from build123d import *

# Parameters (mm, degrees)
SKETCH2_R           = 3.175
BOSS_EXTRUDE1_DEPTH = 57.15
SKETCH7_W           = 12.7
SKETCH7_H           = 15.875
CUT_EXTRUDE3_DEPTH  = 69.170141008
FILLET1_R           = 2.54


with BuildPart() as part:
    # Sketch2 → Boss-Extrude1 (new, symmetric)
    with BuildSketch(Plane(origin=(0, 0, 0), x_dir=(1, 0, 0), z_dir=(0, 1, 0))):
        with BuildLine():
            Line((-28.575, 6.35), (28.575, 6.35))
            ThreePointArc((28.575, 6.35), (34.925, 0), (28.575, -6.35))
            Line((28.575, -6.35), (-28.575, -6.35))
            ThreePointArc((-28.575, -6.35), (-34.925, 0), (-28.575, 6.35))
        make_face()
        with Locations(Location((28.575, 0, 0), (0, 0, 270))):
            Circle(SKETCH2_R, mode=Mode.SUBTRACT)
        with Locations(Location((-28.575, 0, 0), (0, 0, 270))):
            Circle(SKETCH2_R, mode=Mode.SUBTRACT)
    extrude(amount=BOSS_EXTRUDE1_DEPTH, both=True)

    # Sketch7 → Cut-Extrude3 (cut, through all)
    with BuildSketch(Plane.XY.offset(6.35)):
        with Locations((0, 49.2125)):
            Rectangle(SKETCH7_W, SKETCH7_H)
    extrude(amount=-CUT_EXTRUDE3_DEPTH, mode=Mode.SUBTRACT)

    # Fillet1
    fillet1_edges = [part.edges().sort_by_distance(p)[0] for p in [
        (-6.35, 57.15, 0),
        (6.35, 57.15, 0),
        (6.35, 41.275, 0),
        (-6.35, 41.275, 0),
    ]]
    fillet(fillet1_edges, radius=FILLET1_R)


solid = part.part
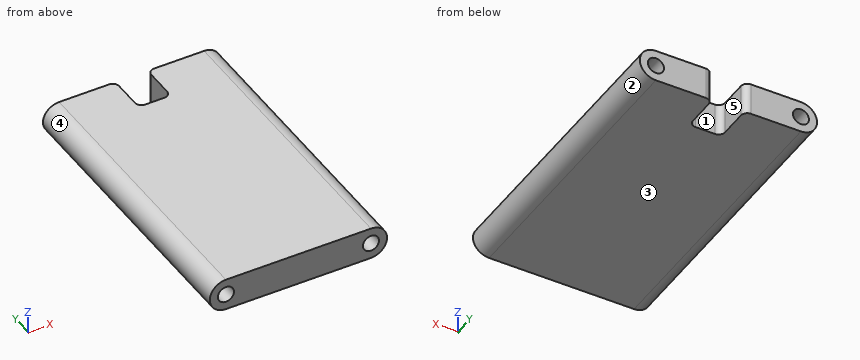
Geometry check sheet. Reference: the model listing, model coordinates, mm. Face numbers are marked on the shaded views. A direction names the side the tool comes from. Coordinates: 2 decimals unless noted, no trailing zeros. Order: outer loops, then holes, each group sorted by start corner. A loop starts at its lowest first (then second) coordinate and runs counter-clockwise, first axis right, second up. Notation, with made-up numbers: (7.25, 34) - (13.25, 34) arc R30 ccw to (13.25, 67) - close; hole circle Ø9 at (-29.75, -17). An arc over 180 degrees is marked (long way). One line per item, written item: value.
(1) Sectioned sample at C-C (z = -5.25). Enter the section's corners in (x, y) (3 decimals).
Data:
outline: (-32.147, -57.15) - (32.147, -57.15) - (32.147, 57.15) - (8.89, 57.15) arc R2.54 ccw to (6.35, 54.61) - (6.35, 43.815) arc R2.54 cw to (3.81, 41.275) - (-3.81, 41.275) arc R2.54 cw to (-6.35, 43.815) - (-6.35, 54.61) arc R2.54 ccw to (-8.89, 57.15) - (-32.147, 57.15) - close
(2) Sectioned sample at B-B (y = 48). Enter the section's corners in (x, z) (3 decimals).
Data:
outline: (-28.575, -6.35) - (-6.35, -6.35) - (-6.35, 6.35) - (-28.575, 6.35) arc R6.35 ccw to start; (6.35, -6.35) - (28.575, -6.35) arc R6.35 ccw to (28.575, 6.35) - (6.35, 6.35) - close; hole circle Ø6.35 at (-28.575, 0); hole circle Ø6.35 at (28.575, 0)
(3) Access from +Z, -Z, +X, -X, +Y, -Y to the whole of each face (thin tool, end or side, straight path). Record for the marked faces 4 and 5.
Data:
face 4: -X, +Y, -Y
face 5: +Z, -Z, +Y
(4) Thickness scan on probe 1 along X at (y, z) = (0.5, 0) (3 decimals); probe 2 along X at (y, z) = (-20.5, -1); probe 3 along X at (y, z) = (49, -5.5). Record the ranges inside material, lowest first. Write a range as from..to.
Data:
probe 1: x = -34.925..-31.75, -25.4..25.4, 31.75..34.925
probe 2: x = -34.85..-31.59, -25.56..25.56, 31.59..34.85
probe 3: x = -31.75..-6.35, 6.35..31.75
(5) Release check for a two-part mould opening along X. For the marked faces 1, 2 and 3 record: +X half, -X half, draft (parallel to the pull), parting line (faces both ways), or undercut.
Data:
face 1: undercut
face 2: +X half
face 3: draft
(6) Depth check by flat-ended pin: pin 1 Ø2.5 at (x, z) = (-2, 0.5) entering from +Y (3 decimals); pin 2 Ø4 at (y, z) = (34, 4) entering from +X; pin 3 Ø1.5 at (y, z) = (5, -3) entering from +X. Enter the tip coordinate at first touch or a pass-through.
Data:
pin 1: stops at y = 41.275
pin 2: stops at x = 34.6
pin 3: stops at x = 34.51
(7) Sectioned sample at A-A (z = 0). Enter the section's corners in (x, y) (3 decimals).
Data:
outline: (-34.925, -57.15) - (-31.75, -57.15) - (-31.75, 57.15) - (-34.925, 57.15) - close; (-25.4, -57.15) - (25.4, -57.15) - (25.4, 57.15) - (8.89, 57.15) arc R2.54 ccw to (6.35, 54.61) - (6.35, 43.815) arc R2.54 cw to (3.81, 41.275) - (-3.81, 41.275) arc R2.54 cw to (-6.35, 43.815) - (-6.35, 54.61) arc R2.54 ccw to (-8.89, 57.15) - (-25.4, 57.15) - close; (31.75, -57.15) - (34.925, -57.15) - (34.925, 57.15) - (31.75, 57.15) - close
